```python
from build123d import *

# Parameters (mm, degrees)
SKETCH1_W           = 55
SKETCH1_H           = 25
BOSS_EXTRUDE1_DEPTH = 3
SKETCH2_R           = 8
CUT_EXTRUDE1_DEPTH  = 3
SKETCH3_W           = 3
SKETCH3_H           = 4
CUT_EXTRUDE2_DEPTH  = 3
SKETCH4_W           = 3
SKETCH4_H           = 4
CUT_EXTRUDE3_DEPTH  = 3
SKETCH5_W           = 5
SKETCH5_H           = 1.5
CUT_EXTRUDE4_DEPTH  = 10


with BuildPart() as part:
    # Sketch1 → Boss-Extrude1 (new body)
    with BuildSketch(Plane.XY):
        Rectangle(SKETCH1_W, SKETCH1_H)
    extrude(amount=BOSS_EXTRUDE1_DEPTH)

    # Sketch2 → Cut-Extrude1 (cut)
    with BuildSketch(Plane.XY.offset(3)):
        with Locations((-13.5, 0)):
            Circle(SKETCH2_R)
        with Locations((13.5, 0)):
            Circle(SKETCH2_R)
    extrude(amount=-CUT_EXTRUDE1_DEPTH, mode=Mode.SUBTRACT)

    # Sketch3 → Cut-Extrude2 (cut)
    with BuildSketch(Plane.XY.offset(3)):
        with Locations((-26, 7.5)):
            Rectangle(SKETCH3_W, SKETCH3_H)
        with Locations((-26, 0.5)):
            Rectangle(SKETCH3_W, SKETCH3_H)
        with Locations((-26, -6.5)):
            Rectangle(SKETCH3_W, SKETCH3_H)
    extrude(amount=-CUT_EXTRUDE2_DEPTH, mode=Mode.SUBTRACT)

    # Sketch4 → Cut-Extrude3 (cut)
    with BuildSketch(Plane.XY.offset(3)):
        with Locations((26, 7.5)):
            Rectangle(SKETCH4_W, SKETCH4_H)
        with Locations((26, 0.5)):
            Rectangle(SKETCH4_W, SKETCH4_H)
        with Locations((26, -6.5)):
            Rectangle(SKETCH4_W, SKETCH4_H)
    extrude(amount=-CUT_EXTRUDE3_DEPTH, mode=Mode.SUBTRACT)

    # Sketch5 → Cut-Extrude4 (cut)
    with BuildSketch(Plane.XY.offset(3)):
        with Locations((0, 11.75)):
            Rectangle(SKETCH5_W, SKETCH5_H)
    extrude(amount=-CUT_EXTRUDE4_DEPTH, mode=Mode.SUBTRACT)


solid = part.part
```
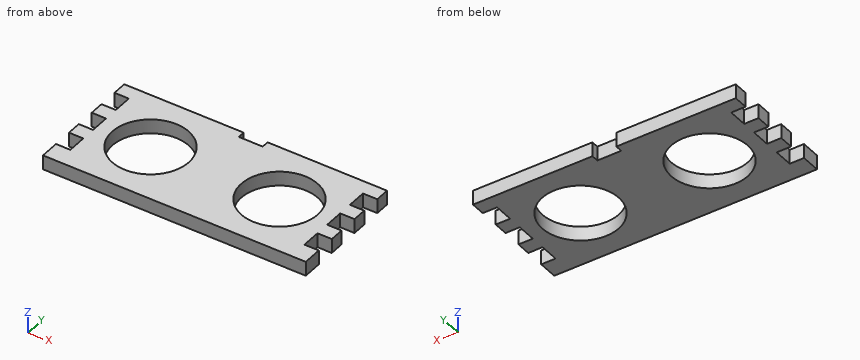
For this review, take the finished solid that the model builds, in its own axes (mm). Round coordinates to 2 decimals unless told otherwise and drop trailing zeros. Write each loop counter-clockwise with the first axis right and the second up, starting at its lowest first coordinate (ties: lowest second). Pieces come first, ordered by that corner, then holes. Notation, with made-up numbers: M -28,66.5 L 17,66.5 A10 cw 17,79.5 Z; hole C 32,70 d2. An arc over 180 degrees is marked long. One line per item, written item: value. Start each with the question number.
(1) We need section A-A (x = -13.5). Give the boundary of the cut face in (y, z).
(2) We need section C-C (z = 0.65). Count the separate pieces of the cut face and the enclosed holes in it, and give its area (3 significant figures).
(3) We need section B-B (y = 0). Give the boundary of the cut face in (x, z), and give its area (3 significant figures).
(4) We need section D-D (y = 9). Give the boundary of the cut face in (x, z), and give its area (3 significant figures).
(5) Wall thickness on line 1 (Y direction, x = 25, z = 1.9); line 2 (X direction, y = -0.25, z = 1.1); line 3 (Y direction, x = -13.5, z = 0.9): over which ranges is each line inside the solid? List them lowest first.
(6) Insertion check: pin 1 (1.5 mm diameter, centred on y = 2, z = 2, fed in from +X); pin 2 (1.5 mm diameter, centred on y = -0.5, z = 2.5, fed in from +X); pin 3 (0.9 mm diameter, centred on y = -6, z = 1, fed in from -X). Each pin has a flat end and moves straight along its axis. Give the tip position at first contact, or say it passes through.
Result:
1. outline: M -12.5,0 L -8,0 L -8,3 L -12.5,3 Z; M 8,0 L 12.5,0 L 12.5,3 L 8,3 Z
2. separate pieces: 1
2. enclosed holes: 2
2. area: 893 mm²
3. outline: M -24.5,0 L -21.5,0 L -21.5,3 L -24.5,3 Z; M -5.5,0 L 5.5,0 L 5.5,3 L -5.5,3 Z; M 21.5,0 L 24.5,0 L 24.5,3 L 21.5,3 Z
3. area: 51.0 mm²
4. outline: M -24.5,0 L 24.5,0 L 24.5,3 L -24.5,3 Z
4. area: 147 mm²
5. line 1: -12.5 to -8.5, -4.5 to -1.5, 2.5 to 5.5, 9.5 to 12.5
5. line 2: -24.5 to -21.5, -5.5 to 5.5, 21.5 to 24.5
5. line 3: -12.5 to -8, 8 to 12.5
6. pin 1: x = 27.5
6. pin 2: x = 24.5
6. pin 3: x = -24.5
